```python
from build123d import *

# Parameters (mm, degrees)
F0_W     = 228.6
F0_H     = 203.2
F0_W_2   = 152.4
F0_H_2   = 152.4
F1_DEPTH = 6.35
F2_W     = 50.8
F2_H     = 6.35
F2_W_2   = 6.35
F2_H_2   = 38.1
F3_DEPTH = 6.35


with BuildPart() as f1:
    # F0 (on Top) → F1 (new body)
    with BuildSketch(Plane.XY):
        with Locations((25.4, 0)):
            Rectangle(F0_W, F0_H)
        Rectangle(F0_W_2, F0_H_2, mode=Mode.SUBTRACT)
    extrude(amount=F1_DEPTH)

    # F2 (on face) → F3 (join)
    with BuildSketch(Plane.XY.offset(6.35)):
        with Locations((-31.75, 104.775)):
            Rectangle(F2_W, F2_H)
        with Locations((82.55, 104.775)):
            Rectangle(F2_W, F2_H)
        with Locations((142.875, 50.8)):
            Rectangle(F2_W_2, F2_H_2)
        with Locations((142.875, -50.8)):
            Rectangle(F2_W_2, F2_H_2)
        with Locations((-92.075, -50.8)):
            Rectangle(F2_W_2, F2_H_2)
        with Locations((-92.075, 50.8)):
            Rectangle(F2_W_2, F2_H_2)
        with Locations((82.55, -104.775)):
            Rectangle(F2_W, F2_H)
        with Locations((-31.75, -104.775)):
            Rectangle(F2_W, F2_H)
    extrude(amount=-F3_DEPTH)


solid = f1.part
```
Could you check a few things on this model? Use its own coordinates, in mm. A direction names the side the tool comes from. Round coordinates to 2 decimals unless told otherwise and drop trailing zeros. Order: outer loops, then holes, each group sorted by start corner. A loop starts at its lowest first (then second) coordinate and runs counter-clockwise, first axis right, second up. Notation, with made-up numbers: M 63,46 L 80,46 A22 cw 80,56 Z; hole C 15,-7 d11. An arc over 180 degrees is marked long. One line per question, with ' | ' between items. Start each with the question number.
(1) Suppose I cut it at A-A on y = -47. List the corners of the cut face in (x, z) for me, then the cut area to 3 significant figures.
(2) Suppose I cut it at C-C on y = -87. List the corners of the cut face in (x, z) for me, then the cut area to 3 significant figures.
(3) For P1, Ø1.9, axis at y = -5.5, z = 4, coming from the +X side; P2, Ø3, axis at y = 106, z = 2, coming from the -X side; P3, Ø3, axis at x = -91.5, z = 2, coming from the +Y side, each with a flat end and sliding along its axis, tell me the tip position at first contact or that it passes through.
(4) For faces 1 (the face through (-88.9, 86, 3)), 2 (the face through (139.7, 86, 3)), 3 (the face through (-88.9, -86, 3)), 4 (the face through (124, -101.6, 3)), which set-ups out of +Z, -Z, +X, -X, +Y, -Y let a thin tool reach every point of the face, with its end or its side?
(5) Please list where these lines run through material, in increasing order: line 1 along X through (y, z) = (31.5, 3.25); line 2 along Y through (x, z) = (-35, 5.5); line 3 along X through (y, z) = (-69.5, 3).
(6) Thinking about a two-plate mould opening in Y: for faces 5 (the face through (-76.2, -1, 3)), 6 (the face through (-57.15, -105, 3)), 7 (the face through (-92, 69.85, 3)), 8 (the face through (-73, -101.6, 3)), which applies, +Y half, -Y half, draft (parallel to the pull), parting line (faces both ways), or undercut?
(7) Suppose I cut it at D-D on x = 116. List the corners of the cut face in (y, z) for me, then the cut area to 3 significant figures.
(8) Suppose I cut it at B-B on x = -64. List the corners of the cut face in (y, z) for me, then the cut area to 3 significant figures.
Geometry results:
1) outline: M -95.25,0 L -76.2,0 L -76.2,6.35 L -95.25,6.35 Z; M 76.2,0 L 146.05,0 L 146.05,6.35 L 76.2,6.35 Z | area: 565 mm²
2) outline: M -88.9,0 L 139.7,0 L 139.7,6.35 L -88.9,6.35 Z | area: 1,450 mm²
3) P1: x = 139.7 | P2: x = -57.15 | P3: y = 69.85
4) face 1: +Z, -Z, -X, +Y | face 2: +Z, -Z, +X, +Y | face 3: +Z, -Z, -X, -Y | face 4: +Z, -Z, +X, -Y
5) line 1: -88.9 to -76.2, 76.2 to 139.7 | line 2: -107.95 to -76.2, 76.2 to 107.95 | line 3: -95.25 to -76.2, 76.2 to 146.05
6) face 5: undercut | face 6: draft | face 7: +Y half | face 8: -Y half
7) outline: M -101.6,0 L 101.6,0 L 101.6,6.35 L -101.6,6.35 Z | area: 1,290 mm²
8) outline: M -101.6,0 L -76.2,0 L -76.2,6.35 L -101.6,6.35 Z; M 76.2,0 L 101.6,0 L 101.6,6.35 L 76.2,6.35 Z | area: 323 mm²
